Build history of the part. All positions in model axes, mm. Give positions to 0.01 mm unless a question says otherwise; leave off trailing zeros. Loops run counter-clockwise (first coordinate to the right, second up) from the corner with the lowest first, then second, coordinate; pieces in that order, holes last. Notation, with made-up numbers: (-19.75, 42) - (20.25, 42) arc R24 ccw to (20.25, 63) - close; hole circle Ø11 at (-23, -7.75). An arc over 180 degrees is marked (long way). Return JSON: item names as keys, results as strings. Group by question number.
1) Drop flat-ended pins along their axis: pin 1 (1 mm diameter, centred on x = 18.5, y = -25.5, fed in from -Z); pin 2 (0.9 mm diameter, centred on x = -4.5, z = 1, fed in from -Y). Give the stop position or say it passes through.
2) Slice it at C-C (x = -66). List the corners of the cut face in (y, z).
3) Slice it at A-A (x = 0). List the corners of the cut face in (y, z), and give its area (3 significant figures).
4) Slice it at D-D (z = 1.35). Count the separate pieces of the cut face and the enclosed holes in it, and give its area (3 significant figures).
5) Drill centre lines: probe 1 along Y at (x, z) = (-52, 0.45); probe 2 along Y at (x, z) = (-0.5, 0.75); probe 3 along X at (y, z) = (46.5, 2.15). Where is each one in solid material? Low to high. Write a range as from..to.
6) Slice it at B-B (y = -11). List the corners of the cut face in (x, z), and give its area (3 significant figures).
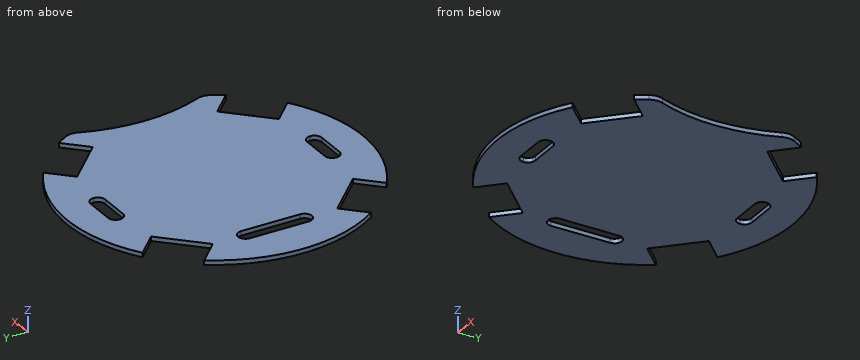
```python
from build123d import *

# Parameters (mm, degrees)
CROQUIS1_R              = 100
SALIENTE_EXTRUIR1_DEPTH = 3
CROQUIS3_R              = 110
CORTAR_EXTRUIR1_DEPTH   = 3
REDONDEO1_R             = 10
CORTAR_EXTRUIR2_DEPTH   = 142.453172607
CROQUIS6_W              = 10
CROQUIS6_H              = 50
CROQUIS6_W_2            = 30
CROQUIS6_H_2            = 10
CORTAR_EXTRUIR4_DEPTH   = 10
REDONDEO3_R             = 5


with BuildPart() as part:
    # Croquis1 → Saliente-Extruir1 (new body)
    with BuildSketch(Plane.XY):
        Circle(CROQUIS1_R)
    extrude(amount=SALIENTE_EXTRUIR1_DEPTH)

    # Croquis3 → Cortar-Extruir1 (cut)
    with BuildSketch(Plane.XY.offset(3)):
        with Locations((190, 0)):
            Circle(CROQUIS3_R)
    extrude(amount=-CORTAR_EXTRUIR1_DEPTH, mode=Mode.SUBTRACT)

    # Redondeo1
    redondeo1_edges = [part.edges().sort_by_distance(p)[0] for p in [
        (89.473684211, -44.659375654, 1.5),
        (89.473684211, 44.659375654, 1.5),
    ]]
    fillet(redondeo1_edges, radius=REDONDEO1_R)

    # Croquis4 → Cortar-Extruir2 (cut, through all)
    with BuildSketch(Plane.XY.offset(3)):
        Polygon((-57.629202667, -83.792153571), (-83.792153571, -57.629202667), (-68.235804385, -42.072853481), (-42.072853481, -68.235804385), align=None)
        Polygon((-57.629202667, 83.792153571), (-42.072853481, 68.235804385), (-68.235804385, 42.072853481), (-83.792153571, 57.629202667), align=None)
        Polygon((83.792153571, 57.629202667), (68.235804385, 42.072853481), (42.072853481, 68.235804385), (57.629202667, 83.792153571), align=None)
        Polygon((57.629202667, -83.792153571), (42.072853481, -68.235804385), (68.235804385, -42.072853481), (83.792153571, -57.629202667), align=None)
    extrude(amount=-CORTAR_EXTRUIR2_DEPTH, mode=Mode.SUBTRACT)

    # Croquis6 → Cortar-Extruir4 (cut)
    with BuildSketch(Plane.XY.offset(3)):
        with Locations((-68.235804385, 0)):
            Rectangle(CROQUIS6_W, CROQUIS6_H)
        with Locations((0, 73.24)):
            Rectangle(CROQUIS6_W_2, CROQUIS6_H_2)
        with Locations((0, -73.24)):
            Rectangle(CROQUIS6_W_2, CROQUIS6_H_2)
    extrude(amount=-CORTAR_EXTRUIR4_DEPTH, mode=Mode.SUBTRACT)

    # Redondeo3
    redondeo3_edges = [part.edges().sort_by_distance(p)[0] for p in [
        (15, -78.24, 1.5),
        (-15, -78.24, 1.5),
        (15, -68.24, 1.5),
        (-15, -68.24, 1.5),
        (-73.235804385, -25, 1.5),
        (-63.235804385, -25, 1.5),
        (-73.235804385, 25, 1.5),
        (-63.235804385, 25, 1.5),
        (-15, 68.24, 1.5),
        (15, 68.24, 1.5),
        (-15, 78.24, 1.5),
        (15, 78.24, 1.5),
    ]]
    fillet(redondeo3_edges, radius=REDONDEO3_R - 0.0001)  # a hair under: the kernel refuses the full size


solid = part.part
```
Results:
{
 "1": {"pin 1": "z = 0", "pin 2": "y = -99.92"},
 "2": {"outline": "(-44.31, 0) - (-24.47, 0) - (-24.47, 3) - (-44.31, 3) - close; (24.47, 0) - (44.31, 0) - (44.31, 3) - (24.47, 3) - close"},
 "3": {"outline": "(-100, 0) - (-78.24, 0) - (-78.24, 3) - (-100, 3) - close; (-68.24, 0) - (68.24, 0) - (68.24, 3) - (-68.24, 3) - close; (78.24, 0) - (100, 0) - (100, 3) - (78.24, 3) - close", "area": "540 mm2"},
 "4": {"separate pieces": "1", "enclosed holes": "3", "area": "26,000 mm2"},
 "5": {"probe 1": "-85.42..-78.16, -58.31..58.31, 78.16..85.42", "probe 2": "-100..-78.24, -68.24..68.24, 78.24..100", "probe 3": "-88.53..-72.66, -63.81..63.81, 72.66..88.14"},
 "6": {"outline": "(-99.39, 0) - (-73.24, 0) - (-73.24, 3) - (-99.39, 3) - close; (-63.24, 0) - (80.55, 0) - (80.55, 3) - (-63.24, 3) - close", "area": "510 mm2"}
}
